Input: part model. Units: mm. Frame: model coordinates. A direction names the side the tool comes from. Round coordinates to 2 decimals unless told otherwise and drop trailing zeros. Order: outer loops, then holes, each group sorted by start corner. A loop starts at its lowest first (then second) coordinate and runs counter-clockwise, first axis right, second up. Notation, with made-up numbers: M -39,89 L -8,89 A29 cw -8,117 Z; hole C 78.5,-32.75 d1. An arc over 180 degrees is marked long. One line per question, with ' | ' between items.
```python
from build123d import *

# Parameters (mm, degrees)
PAD007_DEPTH        = 96
SKETCH010_R         = 1.6
PAD008_DEPTH        = 1.5
LINEARPATTERN_COUNT = 2
LINEARPATTERN_PITCH = 95.5
FILLET002_R         = 1.4
FILLET003_R         = 0.5
FILLET004_R         = 1.4
FILLET005_R         = 0.5


with BuildPart() as part:
    # Sketch009 (on Face5 of Binder009) → Pad007 (new body)
    with BuildSketch(Plane.XZ.offset(50)):
        Polygon((-60.5, -2), (-50.5, -2), (-50.5, -12), (-52, -12), (-52, -3.5), (-60.5, -3.5), align=None)
    extrude(amount=-PAD007_DEPTH)

    # Sketch010 (on Face7 of Pad007) → Pad008 (join)
    with BuildSketch(Plane.XZ.offset(50)):
        with BuildLine():
            ThreePointArc((-57.59, -3.94), (-61.4, -7.75), (-57.59, -11.56))
            Line((-57.59, -11.56), (-52, -11.56))
            Line((-52, -3.94), (-52, -11.56))
            Line((-57.59, -3.94), (-52, -3.94))
        make_face()
        with Locations((-57.59, -7.75)):
            Circle(SKETCH010_R, mode=Mode.SUBTRACT)
    pad008 = extrude(amount=-PAD008_DEPTH)

    # LinearPattern: Pad008 ×2
    with Locations(*[(0, i * LINEARPATTERN_PITCH, 0) for i in range(1, LINEARPATTERN_COUNT)]):
        add(pad008)

    # Fillet002
    fillet002_edges = [part.edges().sort_by_distance(p)[0] for p in [
        (-50.5, -50, -7),
    ]]
    fillet(fillet002_edges, radius=FILLET002_R)

    # Fillet003
    fillet003_edges = [part.edges().sort_by_distance(p)[0] for p in [
        (-52, -48.5, -7.75),
    ]]
    fillet(fillet003_edges, radius=FILLET003_R)

    # Fillet004
    fillet004_edges = [part.edges().sort_by_distance(p)[0] for p in [
        (-50.5, 46, -7),
    ]]
    fillet(fillet004_edges, radius=FILLET004_R)

    # Fillet005
    fillet005_edges = [part.edges().sort_by_distance(p)[0] for p in [
        (-52, 45.5, -7.75),
    ]]
    fillet(fillet005_edges, radius=FILLET005_R)


solid = part.part
```
Item 1: Section query B-B, the plane y = -38.5. Return loops of the section in (x, z), plus the area to 4 significant figures.
Report:
outline: M -60.5,-3.5 L -52,-3.5 L -52,-12 L -50.5,-12 L -50.5,-2 L -60.5,-2 Z | area: 27.75 mm²
Item 2: Access query for faces 1 (the flat face through (-55, 46, -3.94)), 2 (the flat face through (-56, -48.5, -7)), 3 (the flat face through (-55, 46, -11.56)). Directions: +Z, -Z, +X, -X, +Y, -Y. A direction counts if a zero-diameter tool reaches every point of the face in a straight line with its end or side. Return the directions, or none.
Report:
face 1: -X, +Y, -Y | face 2: -Z, -X | face 3: -Z, -X, +Y, -Y
Item 3: Section query A-A, the plane z = -7.75. Return loops of the section in (x, y), plus the area to 3 significant figures.
Report:
outline: M -61.4,-50 L -59.19,-50 L -59.19,-48.5 L -61.4,-48.5 Z; M -61.4,45.5 L -59.19,45.5 L -59.19,47 L -61.4,47 Z; M -55.99,-50 L -51.9,-50 A1.4 ccw -50.5,-48.6 L -50.5,44.6 A1.4 ccw -51.9,46 L -52,46 L -52,47 L -55.99,47 L -55.99,45.5 L -52.5,45.5 A0.5 cw -52,45 L -52,-48 A0.5 cw -52.5,-48.5 L -55.99,-48.5 Z | area: 162 mm²
Item 4: Line query: line 1 along Y through (x, z) = (-56, -9.25); line 2 along Z through (x, y) = (-57.59, -49.1); line 3 along Z through (x, y) = (-57.59, 46.55). Output: solid intervals per line, ascending. Write a range as from..to.
Report:
line 1: -50..-48.5, 45.5..47 | line 2: -11.56..-9.35, -6.15..-3.94, -3.5..-2 | line 3: -11.56..-9.35, -6.15..-3.94
Item 5: Mould query, pull axis Y, two halves, no side actions, for faces 4 (the flat face through (-56, -50, -7)), 5 (the flat face through (-56, -3, -2)), 6 (the flat face through (-56, 45.5, -7)), 7 (the flat face through (-56, 46, -3)). Classes: +Y half, -Y half, draft (parallel to the pull), parting line (faces both ways), or undercut.
Report:
face 4: -Y half | face 5: draft | face 6: undercut | face 7: +Y half
Item 6: First-contact query: pin 1 (1.9 mm diameter, centred on x = -57.59, z = -7.75, fed in from +Y); pin 2 (1.6 mm diameter, centred on x = -55, y = 45.5, fed in from -Z); pin 3 (1 mm diameter, centred on y = -35, z = -7.5, fed in from -X); pin 4 (1.6 mm diameter, centred on y = -20, z = -2.5, fed in from -X). Flat tips, straight axial feed; report the tip coordinate or a pass-through.
Report:
pin 1: through | pin 2: z = -11.56 | pin 3: x = -52 | pin 4: x = -60.5
